```python
from build123d import *

# Parameters (mm, degrees)
SKETCH1_W                            = 126
SKETCH1_H                            = 200
SKETCH1_W_2                          = 106
SKETCH1_H_2                          = 180
RECTANGLE_RIB_DEPTH                  = 1.5
TRIANGLE_RIB_DEPTH                   = 3
M4_CLEARANCE_HOLE1_D                 = 4.8
MIRROR1_AT_THE_SECOND_PLANE_COPY_1_D = 4.8


with BuildPart() as part:
    # Sketch1 → Rectangle Rib (new, symmetric)
    with BuildSketch(Plane.XY):
        Rectangle(SKETCH1_W, SKETCH1_H)
        Rectangle(SKETCH1_W_2, SKETCH1_H_2, mode=Mode.SUBTRACT)
    extrude(amount=RECTANGLE_RIB_DEPTH, both=True)

    # Sketch2 → Triangle Rib (add)
    with BuildSketch(Plane.XY.offset(1.5)):
        Polygon((-63, 100), (0, 235.103935992), (63, 100), (51.96622081, 100), (0, 211.441920161), (-51.96622081, 100), align=None)
    extrude(amount=-TRIANGLE_RIB_DEPTH)

    # M4 Clearance Hole1 (through all)
    with Locations(Plane.XY.offset(1.5)):
        with Locations((-58, 75)):
            m4_clearance_hole1 = Hole(M4_CLEARANCE_HOLE1_D / 2)

    # Mirror1: M4 Clearance Hole1 across plane
    add(m4_clearance_hole1.mirror(Plane.ZX), mode=Mode.SUBTRACT)

    # Mirror1 at the second plane: M4 Clearance Hole1 across plane
    add(m4_clearance_hole1.mirror(Plane(origin=(0, 0, 0), x_dir=(0, 0, 1), z_dir=(1, 0, 0))), mode=Mode.SUBTRACT)

    # Mirror1 at the second plane copy 1 (through all)
    with Locations(Plane(origin=(0, 0, 1.5), x_dir=(-1, 0, 0), z_dir=(0, 0, 1))):
        with Locations((-58, 75)):
            Hole(MIRROR1_AT_THE_SECOND_PLANE_COPY_1_D / 2)


solid = part.part
```
Work out the finished part from the listing and answer in its coordinate system (mm). A direction names the side the tool comes from. Coordinates: 2 decimals unless noted, no trailing zeros. Write each loop counter-clockwise with the first axis right and the second up, starting at its lowest first coordinate (ties: lowest second). Pieces come first, ordered by that corner, then holes. Notation, with made-up numbers: (33.5, -1) - (66.5, -1) arc R29 cw to (66.5, 24) - close; hole circle Ø5 at (44.5, 36.25). An arc over 180 degrees is marked (long way). Answer as a JSON object with one key per item and string values.
Q1. Find section D-D (y = 203.5). Write down the section's boundary in (x, z), plus the area to 3 significant figures.
Results list:
{"outline": "(-14.74, -1.5) - (-3.7, -1.5) - (-3.7, 1.5) - (-14.74, 1.5) - close; (3.7, -1.5) - (14.74, -1.5) - (14.74, 1.5) - (3.7, 1.5) - close", "area": "66.2 mm^2"}
Q2. Find section B-B (z = -0.5). Write down the section's boundary in (x, y), plus the area to 3 significant figures.
Results list:
{"outline": "(-63, -100) - (63, -100) - (63, 100) - (0, 235.1) - (-63, 100) - close; hole circle Ø4.8 at (-58, -75); hole circle Ø4.8 at (-58, 75); hole (-53, -90) - (53, -90) - (53, 90) - (-53, 90) - close; hole (-51.97, 100) - (51.97, 100) - (0, 211.44) - close; hole circle Ø4.8 at (58, -75); hole circle Ø4.8 at (58, 75)", "area": "8,770 mm^2"}
Q3. Given pin 1 Ø4 at (x, y) = (58, -75) entering from +Z, flat-ended and moving along its own axis, determine where the tip first touches the part or whether it passes through.
Results list:
{"pin 1": "passes through"}
Q4. Which of the six approach directions +Z, -Z, +X, -X, +Y, -Y give full straight-line access (tool end or side, diameter ignored) to faces 1 (the flat face through (-31.94, 166.61, 0.02)), 2 (the flat face through (-25.62, 156.5, 0.02))?
Results list:
{"face 1": "+Z, -Z, -X, +Y", "face 2": "+Z, -Z"}
Q5. For a pull along Y with two mould halves and no side action, classify faces 3 (the flat face through (26.347, 154.941, 0.021)), 4 (the flat face through (-4, 93, 1.5)), 5 (the flat face through (31.06, 168.5, 0.02)) as pulls with the +Y half, pulls with the -Y half, needs draft (parallel to the pull), parting line crosses it, or undercut.
Results list:
{"face 3": "undercut", "face 4": "needs draft", "face 5": "pulls with the +Y half"}
Q6. Find section A-A (y = 24). Write down the section's boundary in (x, z), plus the area to 3 significant figures.
Results list:
{"outline": "(-63, -1.5) - (-53, -1.5) - (-53, 1.5) - (-63, 1.5) - close; (53, -1.5) - (63, -1.5) - (63, 1.5) - (53, 1.5) - close", "area": "60.0 mm^2"}
Q7. Consider L1, parallel to X at y = -74.5, z = 1.15; L2, parallel to Y at x = 10.5, z = 0.9; L3, parallel to Y at x = 8.5, z = 1.25. Determine where each line is inside the solid, lowest interval first. Write a range as from..to.
Results list:
{"L1": "x = -63..-60.35, -55.65..-53, 53..55.65, 60.35..63", "L2": "y = -100..-90, 90..100, 188.92..212.59", "L3": "y = -100..-90, 90..100, 193.21..216.88"}
Q8. Find section C-C (x = 44). Write down the section's boundary in (y, z), plus the area to 3 significant figures.
Results list:
{"outline": "(-100, -1.5) - (-90, -1.5) - (-90, 1.5) - (-100, 1.5) - close; (90, -1.5) - (100, -1.5) - (100, 1.5) - (90, 1.5) - close; (117.08, -1.5) - (140.75, -1.5) - (140.75, 1.5) - (117.08, 1.5) - close", "area": "131 mm^2"}
